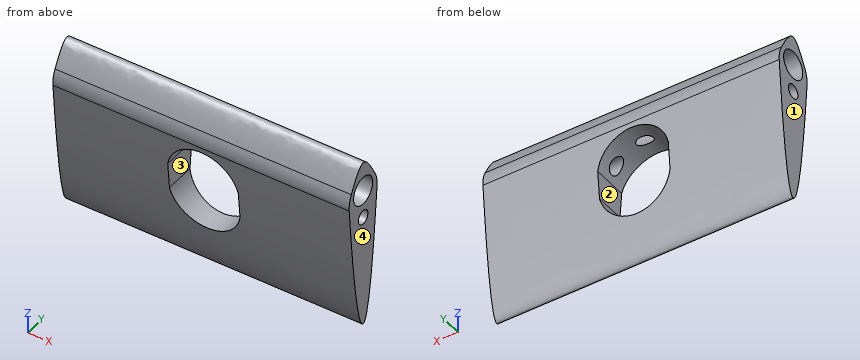
from build123d import *

# Parameters (mm, degrees)
SKETCH1_R               = 5
SKETCH1_R_2             = 2.5
BOSS_EXTRUDE1_DEPTH     = 105
FILLET1_R               = 10
CUT_EXTRUDE1_DEPTH      = 117.542660484
CUT_EXTRUDE1_DEPTH_BACK = 117.542660484


with BuildPart() as part:
    # Sketch1 → Boss-Extrude1 (new body)
    with BuildSketch(Plane(origin=(0, 0, 0), x_dir=(0, 0, -1), z_dir=(1, 0, 0))):
        with BuildLine():
            add(Edge.make_bspline(
                [(3.73e-07, 7.5), (-15, 0), (-3.73e-07, -7.5)],
                knots=[0, 0, 0, 1, 1, 1], degree=2, weights=[1, 2.333333333, 1]))
            add(Edge.make_bspline(
                [(3.73e-07, 7.5), (100, 0), (-3.73e-07, -7.5)],
                knots=[0, 0, 0, 1, 1, 1], degree=2, weights=[1, 1.001467765, 1]))
        make_face()
        Circle(SKETCH1_R, mode=Mode.SUBTRACT)
        with Locations((10, 0)):
            Circle(SKETCH1_R_2, mode=Mode.SUBTRACT)
    extrude(amount=BOSS_EXTRUDE1_DEPTH)

    # Fillet1
    fillet1_edges = [part.edges().sort_by_distance(p)[0] for p in [
        (52.5, 7.5, -3.73e-07),
        (52.5, -7.5, 3.73e-07),
    ]]
    fillet(fillet1_edges, radius=FILLET1_R)

    # Sketch2 → Cut-Extrude1 (cut, two sides)
    with BuildSketch(Plane(origin=(0, 0, 0), x_dir=(1, 0, 0), z_dir=(0, 1, 0))) as cut_extrude1_sk:
        with BuildLine():
            ThreePointArc((65, 24.578179161), (52.5, 34.902500415), (40, 24.578179161))
            Line((40, 24.578179161), (40, 19.76833361))
            Line((40, 19.76833361), (40, 14.958488059))
            ThreePointArc((40, 14.958488059), (52.5, 4.634166805), (65, 14.958488059))
            Line((65, 14.958488059), (65, 19.76833361))
            Line((65, 19.76833361), (65, 24.578179161))
        make_face()
    extrude(amount=CUT_EXTRUDE1_DEPTH, mode=Mode.SUBTRACT)
    extrude(cut_extrude1_sk.sketch, amount=-CUT_EXTRUDE1_DEPTH_BACK, mode=Mode.SUBTRACT)


solid = part.part
For this review, take the finished solid that the model builds, in its own axes (mm). Face numbers are marked on the shaded views. A direction names the side the tool comes from. Round coordinates to 2 decimals unless told otherwise and drop trailing zeros. Put each result on its own line as item: value. Start each with the question number.
1. Insertion check: P1, Ø3, axis at x = 34.5, z = -25.5, coming from the +Y side; P2, Ø6, axis at x = 58, y = -4.5, coming from the +Z side; P3, Ø3, axis at y = 0, z = -10, coming from the -X side; P4, Ø4, axis at x = 22, y = -3, coming from the -Z side. Each pin has a flat end and moves straight along its axis. Give the tip position at first contact, or say it passes through.
2. For the marked faces 3 and 4, list the 3-axis set-ups (+Z, -Z, +X, -X, +Y, -Y) from which the entire face can be reached by the end or side of a thin tool; tool diameter is ignored.
3. Mouldability with a two-part tool opening along Z and no side actions: class the marked faces 1 and 2 as +Z half, -Z half, draft (parallel to the pull), parting line (faces both ways), or undercut.
4. Consider section A-A on y = 0. State how many separate pieces and enclosed holes the cut face has, plus the area to 3 significant figures.
5. For probe 1 along X at (y, z) = (4.5, -17); probe 2 along Z at (x, y) = (8, -0.25); probe 3 along Z at (x, y) = (48.5, 0.75), list the stretches that pass through material, from the lowest coordinate up. Write a range as [from, to].
Result sheet:
1. P1: y = 5.41
1. P2: z = 9.83
1. P3: through
1. P4: z = -49.15
2. face 3: +Y, -Y
2. face 4: +Z, -Z, +X, +Y, -Y
3. face 1: draft
3. face 2: undercut
4. separate pieces: 4
4. enclosed holes: 0
4. area: 4,260 mm^2
5. probe 1: [0, 40], [65, 105]
5. probe 2: [-49.98, -12.49], [-7.51, -4.99], [4.99, 10.48]
5. probe 3: [-49.54, -34.26], [-5.28, -4.94], [4.94, 10.33]
